```python
from build123d import *

# Parameters (mm, degrees)
F0_W      = 120
F0_H      = 150
F1_DEPTH  = 45
F3_DEPTH  = 20
F4_R      = 9
F5_R      = 4
F6_R      = 5
F7_W      = 25.5
F7_H      = 19.05
F8_DEPTH  = 5.1
F10_DEPTH = 3
F12_DEPTH = 22.001


with BuildPart() as f1:
    # F0 (on Front) → F1 (new body)
    with BuildSketch(Plane.XZ):
        with Locations((0, 5)):
            Rectangle(F0_W, F0_H)
    extrude(amount=F1_DEPTH)

    # F2 (on face) → F3 (cut)
    with BuildSketch(Plane.XZ.offset(45)):
        Polygon((-60, -57.6), (60, -57.6), (60, 54.6), (47.3, 80), (-47.3, 80), (-60, 54.6), align=None)
    extrude(amount=-F3_DEPTH, mode=Mode.SUBTRACT)

    # F4
    f4_edges = [f1.edges().sort_by_distance(p)[0] for p in [
        (0, -25, -57.6),
    ]]
    fillet(f4_edges, radius=F4_R)

    # F5
    f5_edges = [f1.edges().sort_by_distance(p)[0] for p in [
        (60, -35, 54.6),
        (-60, -35, 54.6),
        (-47.3, -35, 80),
        (-60, -22.5, 80),
        (60, -22.5, 80),
        (47.3, -35, 80),
    ]]
    fillet(f5_edges, radius=F5_R)

    # F6
    f6_edges = [f1.edges().sort_by_distance(p)[0] for p in [
        (60, -22.5, -70),
        (-60, -22.5, -70),
    ]]
    fillet(f6_edges, radius=F6_R)

    # F7 (on face) → F8 (cut)
    with BuildSketch(Plane(origin=(0, 0, 0), x_dir=(-1, 0, 0), z_dir=(0, 1, 0))):
        with Locations((-0.05, 0)):
            Rectangle(F7_W, F7_H)
        with BuildLine():
            add(Edge.make_bspline(
                [(-3.074624, 33.516029), (-7.791336, 40.77913), (-19.271044, 28.161035), (-30.750752, 15.542941), (-14.554332, 20.897935), (1.642089, 26.252929), (-3.074624, 33.516029)],
                knots=[0, 0, 0, 2.094395, 2.094395, 4.18879, 4.18879, 6.283185, 6.283185, 6.283185], degree=2, weights=[1, 0.5, 1, 0.5, 1, 0.5, 1]))
        make_face()
    extrude(amount=-F8_DEPTH, mode=Mode.SUBTRACT)

    # F9 (on face) → F10 (cut)
    with BuildSketch(Plane.XZ.offset(25)):
        with BuildLine():
            Line((-9.05, 35.9), (-9.05, 33.972442))
            ThreePointArc((-9.05, 33.972442), (0, -14.85), (9.05, 33.972442))
            Line((9.05, 33.972442), (9.05, 35.9))
            Line((9.05, 35.9), (13.05, 35.9))
            Line((13.05, 35.9), (13.05, 40.4))
            Line((13.05, 40.4), (-13.05, 40.4))
            Line((-13.05, 40.4), (-13.05, 35.9))
            Line((-13.05, 35.9), (-9.05, 35.9))
        make_face()
    extrude(amount=-F10_DEPTH, mode=Mode.SUBTRACT)

    # F11 (on face) → F12 (cut, through all)
    with BuildSketch(Plane.XZ.offset(22)):
        Polygon((13.05, 40.4), (-13.05, 40.4), (-13.05, 35.9), (-9.05, 35.9), (9.05, 35.9), (13.05, 35.9), align=None)
    extrude(amount=-F12_DEPTH, mode=Mode.SUBTRACT)


solid = f1.part
```
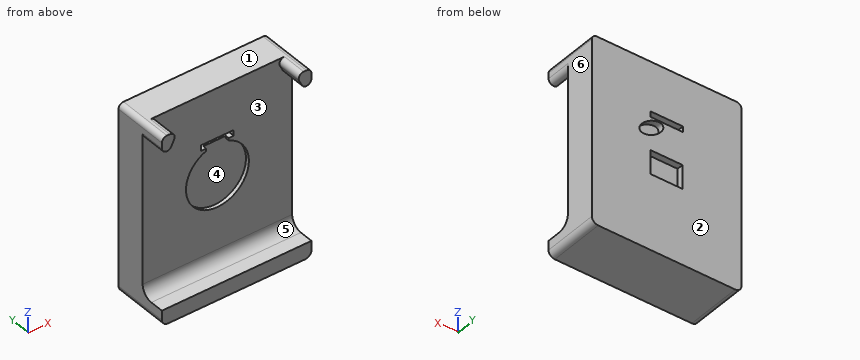
Geometry check sheet. Reference: the model listing, model coordinates, mm. Face numbers are marked on the shaded views. A direction names the side the tool comes from. Give positions to 0.01 mm unless a question says otherwise; leave off trailing zeros. Order: outer loops, then holes, each group sorted by start corner. A loop starts at its lowest first (then second) coordinate and runs counter-clockwise, first axis right, second up.
1. Section check A-A, the plane x = 0. Enter the section's corners in (y, z) (3 decimals).
2. Section check D-D, the plane z = 15. Enter the section's corners in (x, y).
3. Release check for a two-part mould opening along Z. For the marked faces 1, 2, 3 and 4 record: pulls with the +Z half, pulls with the -Z half, needs draft (parallel to the pull), parting line crosses it, or undercut.
4. Thickness scan on L1, parallel to X at y = -24, z = 10; L2, parallel to Z at x = 0, y = -23; L3, parallel to Z at x = -13.5, y = -41. Record the ranges inside material, lowest first.
5. Gauge pin test, flat ends, axial feed: pin 1 Ø3 at (x, y) = (22, -39) entering from +Z; pin 2 Ø7.5 at (x, z) = (11, 26) entering from +Y; pin 3 Ø1 at (x, z) = (28.5, 32.5) entering from -Y. Record the tip position at first contact, or that the pin passes through.
6. Section check B-B, the plane y = -31.5. Enter the section's corners in (x, z).
7. Section check C-C, the plane x = 33. Enter the section's corners in (y, z).
8. Access from +Z, -Z, +X, -X, +Y, -Y to the whole of each face (thin tool, end or side, straight path). Record for the marked faces 5 and 6.
Values follow:
1. outline: (-45, -70) - (0, -70) - (0, -9.525) - (-5.1, -9.525) - (-5.1, 9.525) - (0, 9.525) - (0, 35.9) - (-22, 35.9) - (-22, -14.85) - (-25, -14.85) - (-25, -48.6) arc R9 cw to (-34, -57.6) - (-45, -57.6) - close; (-25, 40.4) - (0, 40.4) - (0, 80) - (-25, 80) - close
2. outline: (-60, -25) - (-24.83, -25) - (-24.83, -22) - (24.83, -22) - (24.83, -25) - (60, -25) - (60, 0) - (-60, 0) - close
3. face 1: pulls with the +Z half
3. face 2: needs draft
3. face 3: undercut
3. face 4: undercut
4. L1: x = -60 to -25.25, 25.25 to 60
4. L2: z = -70 to -14.85, 40.4 to 80
4. L3: z = -70 to -57.6
5. pin 1: stops at z = -57.6
5. pin 2: stops at y = 0
5. pin 3: stops at y = -25
6. outline: (-60, -65) arc R5 ccw to (-55, -70) - (55, -70) arc R5 ccw to (60, -65) - (60, -57.25) - (-60, -57.25) - close; (-60, 71.54) arc R4 ccw to (-52.42, 69.76) - (-50.19, 74.21) arc R4 ccw to (-53.77, 80) - (-56, 80) arc R4 ccw to (-60, 76) - close; (50.19, 74.21) - (52.42, 69.76) arc R4 ccw to (60, 71.54) - (60, 76) arc R4 ccw to (56, 80) - (53.77, 80) arc R4 ccw to start
7. outline: (-45, -70) - (0, -70) - (0, 80) - (-25, 80) - (-25, -48.6) arc R9 cw to (-34, -57.6) - (-45, -57.6) - close
8. face 5: +X, -X, -Y
8. face 6: +Z, -Z, +X, +Y, -Y
